Here's how the part is built. I have some questions about the finished solid (model axes, mm). Face numbers are marked on the shaded views. A direction names the side the tool comes from. Coordinates: 2 decimals unless noted, no trailing zeros. Loops run counter-clockwise (first coordinate to the right, second up) from the corner with the lowest first, then second, coordinate; pieces in that order, holes last. Notation, with made-up numbers: M 6,66 L 44,66 A13 ccw 44,84 Z; hole C 18.5,77.5 d6. An arc over 180 degrees is marked long. Use one line per item in the form item = value. Start each with the question number.
(1) Imagine slicing it at C-C, the plane y = 5.5. Please give me the cut outline in (x, z) (3 decimals).
(2) Thinking about a two-plate mould opening in X: for the marked faces 1, 2 and 3, which applies, +X half, -X half, draft (parallel to the pull), parting line (faces both ways), or undercut?
(3) On a 3-axis mill with a long thin cutter (end or side, diameter ignored), from which of +Z, -Z, +X, -X, +Y, -Y can I reach the whole of each face in a straight line? I mean the marked faces 4 and 5. Say none if no direction works.
(4) Please list where these lines run through material, in increasing order: L1, parallel to X at y = 3.25, z = -2; L2, parallel to Z at x = 16.51, y = 2.4; L3, parallel to Y at x = 5.5, z = -7.5.
(5) Will these pins go through, and if not, where does the flat tip stop? P1, Ø2, axis at y = 11.5, z = -8, coming from the -X side; P2, Ø5, axis at y = 14.5, z = -6.5, coming from the +X side; P3, Ø1.7, axis at x = 16.51, z = -9.525, coming from the -Y side.
(6) Imagine slicing it at B-B, the plane y = 1.75. Please give me the cut outline in (x, z) (3 decimals), and give its area (3 significant figures).
(7) Imagine slicing it at D-D, the plane y = 9.25. Please give me the cut outline in (x, z) (1 decimal), and give its area (3 significant figures).
```python
from build123d import *

# Parameters (mm, degrees)
SKETCH1_W                      = 25.4
SKETCH1_H                      = 11.43
BOSS_EXTRUDE1_DEPTH            = 6.35
SKETCH2_R                      = 4.7625
BOSS_EXTRUDE2_DEPTH            = 9.525
SKETCH3_R                      = 2.4511
CUT_EXTRUDE1_DEPTH             = 33.059640126
F_60_0_04_DIAMETER_HOLE1_D     = 2.8448
F_60_0_04_DIAMETER_HOLE1_DEPTH = 3.96875
F_60_0_04_DIAMETER_HOLE1_TIP   = 0.854664145


with BuildPart() as part:
    # Sketch1 → Boss-Extrude1 (new body)
    with BuildSketch(Plane(origin=(0, 0, 0), x_dir=(1, 0, 0), z_dir=(0, 1, 0))):
        with Locations((12.7, 5.715)):
            Rectangle(SKETCH1_W, SKETCH1_H)
    extrude(amount=BOSS_EXTRUDE1_DEPTH)

    # Sketch2 → Boss-Extrude2 (add)
    with BuildSketch(Plane(origin=(0, 6.35, 0), x_dir=(1, 0, 0), z_dir=(0, 1, 0))):
        with Locations(Location((12.7, 5.715, 0), (0, 0, 90))):
            Circle(SKETCH2_R)
    extrude(amount=BOSS_EXTRUDE2_DEPTH)

    # Sketch3 → Cut-Extrude1 (cut, through all)
    with BuildSketch(Plane(origin=(0, 15.875, 0), x_dir=(1, 0, 0), z_dir=(0, 1, 0))):
        with Locations(Location((12.7, 5.715, 0), (0, 0, 270))):
            Circle(SKETCH3_R)
    extrude(amount=-CUT_EXTRUDE1_DEPTH, mode=Mode.SUBTRACT)

    # #60 (0.04) Diameter Hole1
    with Locations(Plane(origin=(8.89, 0, -1.905), x_dir=(0, 0, -1), z_dir=(0, -1, 0))):
        with Locations((0, 0), (7.62, 0), (7.62, 7.62), (0, 7.62)):
            Hole(F_60_0_04_DIAMETER_HOLE1_D / 2, depth=F_60_0_04_DIAMETER_HOLE1_DEPTH)
            with Locations((0, 0, -(F_60_0_04_DIAMETER_HOLE1_DEPTH + F_60_0_04_DIAMETER_HOLE1_TIP / 2))):  # 118° drill point
                Cone(0, F_60_0_04_DIAMETER_HOLE1_D / 2, F_60_0_04_DIAMETER_HOLE1_TIP, mode=Mode.SUBTRACT)


solid = part.part
```
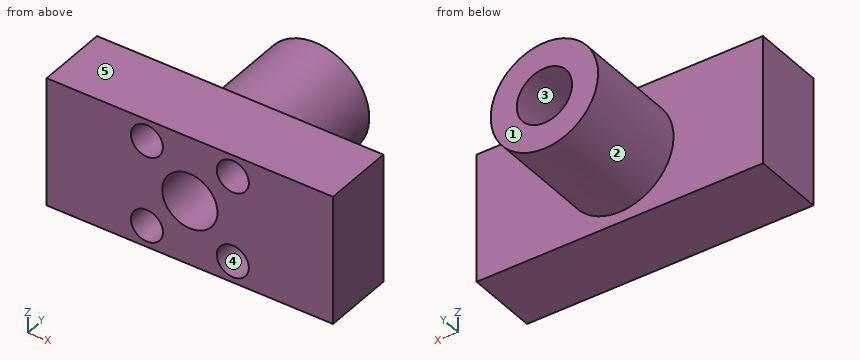
Answer:
q1.outline = M 0,-11.43 L 25.4,-11.43 L 25.4,0 L 0,0 Z; hole C 12.7,-5.715 d4.902
q2.face_1 = draft
q2.face_2 = parting line
q2.face_3 = undercut
q3.face_4 = -Y
q3.face_5 = +Z, +X, -X, +Y, -Y
q4.L1 = 0 to 7.47, 10.31 to 15.09, 17.93 to 25.4
q4.L2 = -11.43 to -10.95, -8.1 to -3.33, -0.48 to 0
q4.L3 = 0 to 6.35
q5.P1 = 8.11
q5.P2 = 17.46
q5.P3 = 4.31
q6.outline = M 0,-11.43 L 25.4,-11.43 L 25.4,0 L 0,0 Z; hole C 8.89,-9.525 d2.845; hole C 8.89,-1.905 d2.845; hole C 12.7,-5.715 d4.902; hole C 16.51,-9.525 d2.845; hole C 16.51,-1.905 d2.845
q6.area = 246 mm²
q7.outline = C 12.7,-5.7 d9.5; hole C 12.7,-5.7 d4.9
q7.area = 52.4 mm²
